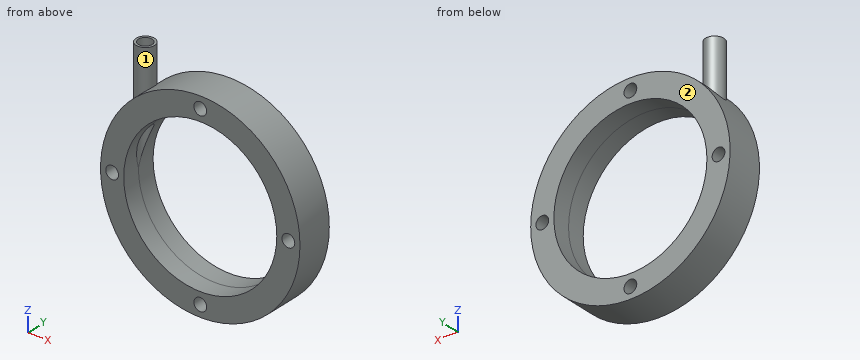
```python
from build123d import *

# Parameters (mm, degrees)
SKETCH001_R           = 43
PAD_DEPTH             = 8
SKETCH002_W           = 4
SKETCH002_H           = 50
SKETCH003_R           = 33
POCKET_DEPTH          = 8.001
POCKET_DEPTH_BACK     = 8.001
SKETCH004_W           = 3
SKETCH004_H           = 50
SKETCH013_R           = 2.75
POCKET005_DEPTH       = 271.35174
POLARPATTERN003_COUNT = 4


with BuildPart() as part:
    # Sketch001 → Pad (new body, symmetric)
    with BuildSketch(Plane.XZ):
        Circle(SKETCH001_R)
    extrude(amount=PAD_DEPTH, both=True)

    # Sketch002 → Revolution (revolve)
    with BuildSketch(Plane.XZ):
        with Locations((-28, 25)):
            Rectangle(SKETCH002_W, SKETCH002_H)
    revolve(axis=Axis((-30, 0, 40.402922), (0, 0, 1)))

    # Sketch003 → Pocket (cut, two sides)
    with BuildSketch(Plane.XZ) as pocket_sk:
        Circle(SKETCH003_R)
    extrude(amount=-POCKET_DEPTH, mode=Mode.SUBTRACT)
    extrude(pocket_sk.sketch, amount=POCKET_DEPTH_BACK, mode=Mode.SUBTRACT)

    # Sketch004 → Groove (revolve, cut)
    with BuildSketch(Plane.XZ):
        with Locations((-31.5, 25)):
            Rectangle(SKETCH004_W, SKETCH004_H)
    revolve(axis=Axis((-30, 0, 22.276785), (0, 0, 1)), mode=Mode.SUBTRACT)

    # Sketch013 (on Face4 of Groove) → Pocket005 (cut, through all)
    with BuildSketch(Plane.XZ.offset(8)):
        with Locations((38, 0)):
            Circle(SKETCH013_R)
    pocket005 = extrude(amount=-POCKET005_DEPTH, mode=Mode.SUBTRACT)

    # PolarPattern003: Pocket005 ×4 about axis
    polarpattern003_axis = Axis((0, -8, 0), (0, -1, 0))
    for i in range(1, POLARPATTERN003_COUNT):
        add(pocket005.rotate(polarpattern003_axis, i * 360 / POLARPATTERN003_COUNT), mode=Mode.SUBTRACT)


solid = part.part
```
Geometry: final body of the model. Coordinates: model frame, mm. Face numbers are marked on the shaded views. A direction names the side the tool comes from. Coordinates: 2 decimals unless noted, no trailing zeros. Order: outer loops, then holes, each group sorted by start corner. A loop starts at its lowest first (then second) coordinate and runs counter-clockwise, first axis right, second up. Notation, with made-up numbers: (-15, 81) - (35, 81) arc R20 cw to (35, 92) - close; hole circle Ø10 at (60, 53). An arc over 180 degrees is marked (long way). Write each question's results on one line, items separated by ' | '.
1) Line query: line 1 (X direction, y = -0.5, z = 28.5); line 2 (X direction, y = 0, z = 25.5); line 3 (Z direction, x = 3, y = 2.5). Output: solid intervals per line, ascending. Write a range as from..to.
Results list:
line 1: -33.97..-32.96, -27.04..-16.64, 16.64..32.2 | line 2: -34.62..-33, -27..-20.95, 20.95..34.62 | line 3: -42.9..-32.86, 32.86..42.9
2) Section B-B, the plane x = -11. Return loops of the section in (y, z), plus the area to 3 significant figures.
Results list:
outline: (-8, -41.57) - (8, -41.57) - (8, -31.11) - (-8, -31.11) - close; (-8, 31.11) - (8, 31.11) - (8, 41.57) - (-8, 41.57) - close | area: 335 mm^2
3) Pin query (flat end, axial travel): pin 1 (4.5 mm diameter, centred on x = 38, z = 0, fed in from +Y); pin 2 (6 mm diameter, centred on x = 8.5, y = 6, fed in from -Z); pin 3 (2 mm diameter, centred on x = 25.5, y = -4, fed in from +Z); pin 4 (3.5 mm diameter, centred on x = -30, y = 0, fed in from -Z). Return the tip coordinate at first contact, or that it passes through.
Results list:
pin 1: through | pin 2: z = -42.65 | pin 3: z = 35.34 | pin 4: z = -32.42
4) Set-up query: the marked faces 1 and 2. Return all of +Z, -Z, +X, -X, +Y, -Y with unobstructed straight access to the full face (end or side cutting, diameter ignored); none if empty.
Results list:
face 1: +Z | face 2: +Z, -Z, +X, -X, +Y
5) Section D-D, the plane x = -29. Return loops of the section in (y, z).
Results list:
outline: (-8, -31.75) - (8, -31.75) - (8, -15.75) - (-8, -15.75) - close; (-8, 15.75) - (-2.83, 15.75) - (-2.83, 50) - (-3.87, 50) - (-3.87, 31.75) - (-8, 31.75) - close; (2.83, 15.75) - (8, 15.75) - (8, 31.75) - (3.87, 31.75) - (3.87, 50) - (2.83, 50) - close
6) Section C-C, the plane z = -25. Return loops of the section in (x, y).
Results list:
outline: (-34.99, -8) - (-21.54, -8) - (-21.54, 8) - (-34.99, 8) - close; (21.54, -8) - (34.99, -8) - (34.99, 8) - (21.54, 8) - close
7) Section A-A, the plane z = 38. Return loops of the section in (x, y).
Results list:
outline: circle Ø8 at (-30, 0); (-20.12, -8) - (-2.75, -8) - (-2.75, 8) - (-20.12, 8) - close; (2.75, -8) - (20.12, -8) - (20.12, 8) - (2.75, 8) - close; hole circle Ø6 at (-30, 0)
